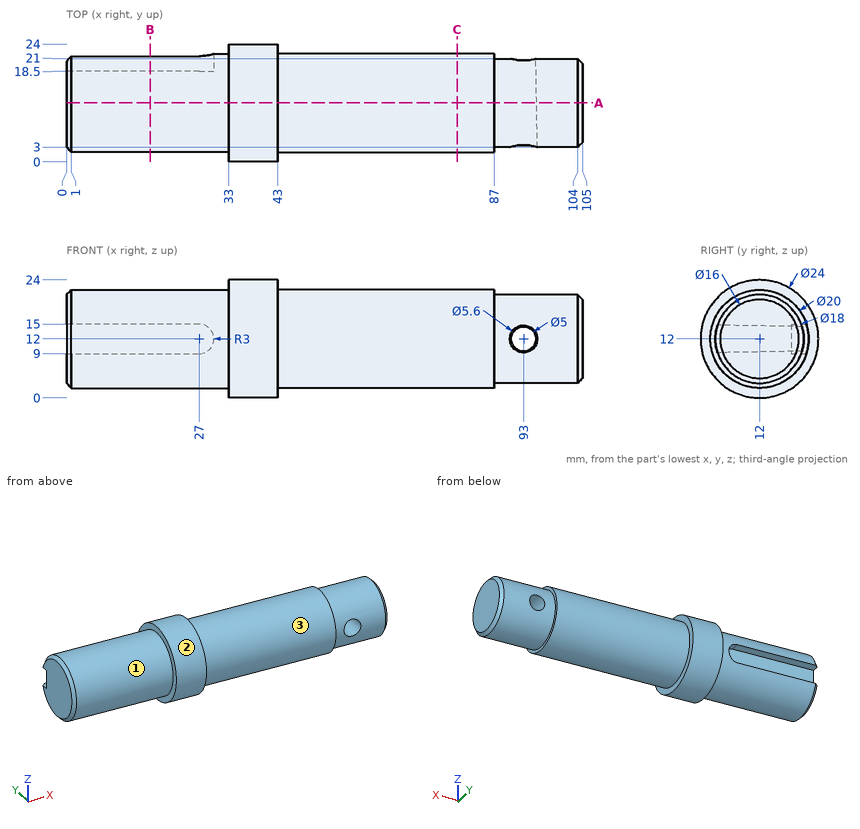
Here's the drawing with two shaded views (mm, measured from the low corner). I have some questions. A direction names the side the tool comes from. Give positions to 0.01 mm unless a question says otherwise; leave off trailing zeros. Loops run counter-clockwise (first coordinate to the right, second up) from the corner with the lowest first, then second, coordinate; pieces in that order, holes last. Notation, with made-up numbers: M 21,0.5 L 62,0.5 A14 ccw 62,8.5 Z; hole C 27,6 d10. An arc over 180 degrees is marked long. Use one line per item in the form item = value. Start each with the question number.
(1) I want a section at B-B, the plane x = 17. Write out the boundary of the cut face in (y, z).
(2) I'm going to push flat-ended pins straight in: P1, Ø0.9, axis at x = 11, y = 20, coming from the -Z side; P2, Ø6, axis at x = 90.5, z = 8.5, coming from the +Y side; P3, Ø12, axis at y = 3.5, z = 18.5, coming from the -X side; P4, Ø4, axis at x = 65.5, z = 5, coming from the -Y side. Where does each tip first touch, or does it pass through?
(3) I want a section at A-A, the plane y = 12. Write out the boundary of the cut face in (x, z).
(4) I want a section at C-C, the plane x = 79.5. Write out the boundary of the cut face in (y, z), and give its area (3 significant figures).
(5) Please list where these lines run through material, in increasing order: line 1 (Z direction, x = 78.5, y = 18); line 2 (X direction, y = 21.75, z = 17.75); line 3 (X direction, y = 17.5, z = 14.25).
(6) On a 3-axis mill with a long thin cutter (end or side, diameter ignored), from which of +Z, -Z, +X, -X, +Y, -Y can I reach the whole of each face in a straight line? I mean the marked faces 1, 2 and 3. Say none if no direction works.
Worked out:
q1.outline = M 18.5,9 L 18.5,15 L 21.54,15 A10 ccw long 21.54,9 Z
q2.P1 = 5.44
q2.P2 = 20.99
q2.P3 = 0
q2.P4 = 3.34
q3.outline = M 0,3 L 1,2 L 33,2 L 33,0 L 43,0 L 43,2 L 87,2 L 87,3 L 104,3 L 105,4 L 105,20 L 104,21 L 87,21 L 87,22 L 43,22 L 43,24 L 33,24 L 33,22 L 1,22 L 0,21 Z; hole C 93,12 d5.3
q4.outline = C 12,12 d20
q4.area = 314 mm²
q5.line_1 = 4 to 20
q5.line_2 = 33 to 43
q5.line_3 = 0 to 91.78, 94.22 to 105
q6.face_1 = -X
q6.face_2 = +X, -X
q6.face_3 = +X
